CAD build for the part. Positions are in the model's coordinates, mm. A direction names the side the tool comes from. Coordinates: 2 decimals unless noted, no trailing zeros. Loops run counter-clockwise (first coordinate to the right, second up) from the corner with the lowest first, then second, coordinate; pieces in that order, holes last. Notation, with made-up numbers: (66, 58.25) -> (106, 58.25) arc R28 cw to (106, 89.25) -> close; hole circle Ø6 at (2.5, 24.5). An arc over 180 degrees is marked (long way). Write item = value, one per line. Start each with the question number.
(1) Pull direction Y, two halves, no side cores. Call faces 1 (the face through (-28.04, 6.07, -27.5)), 2 (the face through (0, 5, -22)), 3 (the face through (-12.8, 8, -22.2)), 4 (the face through (-2, 6, 0)): +Y half, -Y half, draft (parallel to the pull), parting line (faces both ways), or undercut.
(2) Band-saw the part on C-C (x = -24.5). Write the cut outline in (y, z), and give its area (3 significant figures).
(3) Band-saw the part on A-A (z = -31.4). Write the cut outline in (x, y).
(4) Band-saw the part on D-D (y = 6). Write the cut outline in (x, z), and give its area (3 significant figures).
(5) Band-saw the part on B-B (y = 3.5). Write the cut outline in (x, z), and give its area (3 significant figures).
(6) Flat gauge pins, fed straight in: P1, Ø7.5, axis at x = -25.5, z = -30.5, coming from the -Y side; P2, Ø0.9, axis at x = 0, z = -22.5, coming from the -Y side; P3, Ø1.6, axis at x = -27.5, y = 5, coming from the -Z side; P4, Ø3, axis at x = -25, z = -31.4, coming from the -Y side. Where does each tip first touch, or does it go through?
(7) Tool access for faces 5 (the face through (-27, 5, -28)), 6 (the face through (-0.5, 1.5, 0)), 7 (the face through (-21.5, 2, -29)): list every direction of +Z, -Z, +X, -X, +Y, -Y with a clear straight run to the whole face (end or side of a thin tool).
(8) Drill centre lines: line 1 (Z direction, x = -25, y = 1.7); line 2 (X direction, y = 1.55, z = 3); line 3 (Z direction, x = -19.5, y = 4). Where is each one in solid material? Low to high. Write a range as from..to.
Autodesk Inventor part; units mm, degrees
ref_plane "YZ Plane" through (0, 0, 0) normal (1, 0, 0) x (0, 1, 0)
ref_plane "XZ Plane" through (0, 0, 0) normal (0, 1, 0) x (-1, 0, 0)
ref_plane "XY Plane" through (0, 0, 0) normal (0, 0, 1) x (1, 0, 0)
sketch "Szkic1" plane through (0, 0, 0) normal (0, 1, 0) x (-1, 0, 0)
  line L0 (0, 0) -> (3, 0)
  line L1 (3, 0) -> (3, -25)
  line L2 (3, -25) -> (0, -25)
  line L3 (0, -25) -> (0, 0)
  line L4 (3, -25) -> (31, -25)
  line L5 (31, -25) -> (31, -22)
  line L6 (31, -22) -> (3, -22)
  line L7 (3, -22) -> (3, -25)
  point P0 (3, -22)
  dimension "d0" = 3
  dimension "d1" = 25
  dimension "d2" = 28
  dimension "d3" = 3
extrude "Wyciągnięcie proste1" add sketch "Szkic1" along normal blind 8
sketch "Szkic2" plane through (0, 0, 0) normal (1, 0, 0) x (0, 0, -1)
  line L0 (0, 0) -> (0, 8)
  line L1 (0, 8) -> (5, 8)
  line L2 (5, 8) -> (5, 0)
  line L3 (5, 0) -> (0, 0)
  line L4 (0, 0) -> (0, 8)
  dimension "d6" = 5
  dimension "d7" = 8
extrude "Wyciągnięcie proste2" add sketch "Szkic2" along normal blind 3
sketch "Szkic6" plane through (0, 8, 0) normal (0, 1, 0) x (1, 0, 0)
  line L0 (-31, 22) -> (-3, 22)
  line L1 (0, 25) -> (-31, 25)
  line L2 (-3, 22) -> (0, 22)
  line L3 (0, 22) -> (0, 25)
  line L4 (0, 25) -> (-3, 25)
  line L5 (-3, 25) -> (-3, 22)
  line L6 (-3, 25) -> (3, 25)
  line L7 (3, 25) -> (3, 19)
  line L8 (3, 19) -> (-3, 19)
  line L9 (-3, 19) -> (-3, 25)
  point P0 (0, 0)
  dimension "d19" = 6
  dimension "d20" = 6
extrude "Wyciągnięcie proste6" add sketch "Szkic6" against normal blind 8 contours L6 L7 L8 L9 L2 L3
sketch "Szkic7" plane through (0, 8, 0) normal (0, 1, 0) x (1, 0, 0)
  line L0 (3, 19) -> (3, 25)
  line L1 (-31, 25) -> (3, 25)
  line L2 (-3, 22) -> (-3, 0)
  circle A0 centre (0, 22) radius 1.5
  point P0 (0, 0)
  dimension "d23" = 3
  dimension "d42" = 3
  dimension "d43" = 3
extrude "Wyciągnięcie proste7" cut sketch "Szkic7" against normal blind 8
sketch "Szkic8" plane through (0, 8, 0) normal (0, 1, 0) x (1, 0, 0)
  circle A0 centre (0, 22) radius 1.5
  circle A1 centre (0, 22) radius 2
  point P0 (0, 0)
extrude "Wyciągnięcie proste8" add sketch "Szkic8" against normal blind 3 contours A0
sketch "Szkic9" plane through (0, 8, 0) normal (0, 1, 0) x (1, 0, 0)
  line L0 (-31, 25) -> (-31, 22)
  line L1 (3, 19) -> (3, 25)
  line L2 (-31, 25) -> (3, 25)
  line L3 (3, 25) -> (3, 24)
  line L4 (3, 24) -> (-31, 24)
  line L5 (-31, 24) -> (-31, 25)
  point P0 (0, 0)
  dimension "d28" = 1
extrude "Wyciągnięcie proste9" cut sketch "Szkic9" against normal blind 8
sketch "Szkic10" plane through (0, 0, -5) normal (0, 0, -1) x (-1, 0, 0)
  line L0 (0, 0) -> (0, 8)
  line L1 (-3, 8) -> (-3, 0)
  line L2 (0, 0) -> (-3, 0)
  line L3 (-3, 0) -> (-3, 8)
  line L4 (-3, 8) -> (0, 8)
  line L5 (0, 8) -> (0, 0)
  point P0 (-3, 0)
extrude "Wyciągnięcie proste10" cut sketch "Szkic10" against normal blind 3.7
sketch "Szkic11" plane through (0, 8, -19) normal (0, 0, 1) x (1, 0, 0)
  line L0 (-3, 0) -> (3, 0)
  line L1 (3, -8) -> (0, -8)
  line L2 (0, 0) -> (3, 0)
  line L3 (3, 0) -> (3, -8)
  line L4 (3, -8) -> (0, -8)
  line L5 (0, -8) -> (0, 0)
extrude "Wyciągnięcie proste11" cut sketch "Szkic11" against normal blind 0.5
sketch "Szkic12" plane through (3, 8, -24) normal (0, 0, -1) x (-1, 0, 0)
  line L0 (0, -8) -> (0, 0)
  line L1 (6, 0) -> (0, 0)
  line L2 (0, -8) -> (6, -8)
  line L3 (6, -8) -> (6, 0)
  line L4 (6, 0) -> (0, 0)
  line L5 (0, 0) -> (0, -8)
  point P0 (3, -8)
extrude "Wyciągnięcie proste12" add sketch "Szkic12" along normal blind 0.5
sketch "Szkic13" plane through (0, 0, -1.3) normal (1, 0, 0) x (0, 0, -1)
  line L0 (0, 0) -> (18.2, 0)
  line L1 (0, 8) -> (18.2, 8)
  line L2 (0, 0) -> (18.2, 0)
  line L3 (18.2, 0) -> (18.2, 8)
  line L4 (18.2, 8) -> (0, 8)
  line L5 (0, 8) -> (0, 0)
  point P0 (-1.3, 0)
  point P1 (18.2, 0)
extrude "Wyciągnięcie proste13" cut sketch "Szkic13" against normal blind 1
sketch "Szkic14" plane through (3, 8, -24.5) normal (0, 0, -1) x (-1, 0, 0)
  line L0 (4, 0) -> (0, 0)
  line L1 (6, -8) -> (6, 0)
  line L2 (0, 0) -> (6, 0)
  line L3 (6, 0) -> (6, -8)
  line L4 (6, -8) -> (0, -8)
  line L5 (0, -8) -> (0, 0)
  point P0 (3, -8)
extrude "Wyciągnięcie proste14" cut sketch "Szkic14" against normal blind 0.5
sketch "Szkic15" plane through (-3, 0, 0) normal (0, 0, 1) x (1, 0, 0)
  line L0 (6, 8) -> (6, 0)
  line L1 (0, 0) -> (0, 8)
  line L2 (6, 8) -> (0, 8)
  line L3 (0, 8) -> (0, 0)
  line L4 (0, 0) -> (6, 0)
  line L5 (6, 0) -> (6, 8)
  point P0 (3, 0)
extrude "Wyciągnięcie proste15" add sketch "Szkic15" along normal blind 4.7
sketch "Szkic16" plane through (3, 0, 0) normal (1, 0, 0) x (0, 0, -1)
  line L0 (-4.7, 8) -> (-4.7, 0)
  line L1 (1.3, 0) -> (1.3, 8)
  line L2 (-4.7, 0) -> (1.3, 0)
  line L3 (1.3, 0) -> (1.3, 8)
  line L4 (1.3, 8) -> (-4.7, 8)
  line L5 (-4.7, 8) -> (-4.7, 0)
  point P0 (0, 0)
extrude "Wyciągnięcie proste16" cut sketch "Szkic16" against normal blind 4
sketch "Szkic17" plane through (0, 8, 0) normal (0, 1, 0) x (1, 0, 0)
  line L0 (-1, 19.5) -> (-1, -4.7)
  line L1 (-3, -4.7) -> (-1, -4.7)
  line L2 (-1, -4.7) -> (-1, 0)
  line L3 (-1, 0) -> (-3, 0)
  line L4 (-3, 0) -> (-3, -4.7)
  line L5 (-3, 0) -> (3, 0)
  line L6 (3, 0) -> (3, -6)
  line L7 (3, -6) -> (-3, -6)
  line L8 (-3, -6) -> (-3, 0)
  point P0 (0, 0)
  dimension "d48" = 6
  dimension "d49" = 6
extrude "Wyciągnięcie proste17" cut sketch "Szkic17" against normal blind 5
sketch "Szkic18" plane through (0, 3, 0) normal (0, 1, 0) x (1, 0, 0)
  line L0 (-3, 0) -> (-1, 0)
  line L1 (-3, 0) -> (3, 0)
  line L2 (3, 0) -> (3, -6)
  line L3 (3, -6) -> (-3, -6)
  line L4 (-3, -6) -> (-3, 0)
  point P0 (0, 0)
  dimension "d52" = 6
  dimension "d53" = 6
extrude "Wyciągnięcie proste18" add sketch "Szkic18" against normal blind 3
sketch "Szkic19" plane through (0, 3, 0) normal (0, 1, 0) x (1, 0, 0)
  circle A0 centre (0, -3) radius 2
  line L0 (-3, -6) -> (-3, 0)
  line L1 (-3, -6) -> (3, -6)
  point P0 (0, 0)
  dimension "d56" = 4
  dimension "d57" = 3
  dimension "d58" = 3
extrude "Wyciągnięcie proste19" cut sketch "Szkic19" against normal blind 3
sketch "Szkic20" plane through (-31, 0, -22) normal (0, 0, 1) x (1, 0, 0)
  line L0 (34, 8) -> (0, 8)
  line L1 (0, 8) -> (7, 8)
  line L2 (7, 8) -> (7, 4)
  line L3 (7, 4) -> (0, 4)
  line L4 (0, 4) -> (0, 8)
  point P0 (31, 0)
  point P1 (7, 8)
  dimension "d61" = 7
  dimension "d62" = 4
extrude "Wyciągnięcie proste20" add sketch "Szkic20" along normal blind 4
sketch "Szkic21" plane through (-31, 0, -24) normal (-1, 0, 0) x (0, 0, 1)
  circle A0 centre (4, 6) radius 1.5
  line L0 (6, 8) -> (6, 4)
  line L1 (2, 4) -> (6, 4)
  point P0 (24, 0)
  point P1 (4, 4)
  dimension "d65" = 3
  dimension "d66" = 2
  dimension "d67" = 2
extrude "Wyciągnięcie proste21" cut sketch "Szkic21" against normal blind 6
sketch "Szkic22" plane through (3, 8, -24) normal (0, 0, -1) x (-1, 0, 0)
  line L0 (34, 0) -> (34, -8)
  line L1 (34, 0) -> (27, 0)
  line L2 (27, 0) -> (27, -4)
  line L3 (27, -4) -> (34, -4)
  line L4 (34, -4) -> (34, 0)
  point P0 (3, -8)
  dimension "d70" = 7
  dimension "d71" = 4
extrude "Wyciągnięcie proste22" add sketch "Szkic22" along normal blind 4
sketch "Szkic23" plane through (-31, 0, -24) normal (-1, 0, 0) x (0, 0, 1)
  circle A0 centre (-2, 6) radius 1.5
  line L0 (-4, 8) -> (6, 8)
  line L1 (-4, 4) -> (-4, 8)
  line L2 (2, 0) -> (2, 8)
  line L3 (6, 8) -> (2, 8)
  line L4 (2, 8) -> (2, 4)
  line L5 (2, 4) -> (6, 4)
  line L6 (6, 4) -> (6, 8)
  point P0 (24, 0)
  point P1 (-4, 6)
  dimension "d74" = 3
  dimension "d75" = 2
  dimension "d76" = 2
extrude "Wyciągnięcie proste23" cut sketch "Szkic23" against normal blind 7 contours L0 L6 L5 L2
extrude "Wyciągnięcie proste24" cut sketch "Szkic23" against normal blind 6 contours A0
sketch "Sketch24" plane through (3, 0, -24) normal (0, 0, -1) x (-1, 0, 0)
  line L0 (34, 4) -> (27, 4)
  line L1 (27, 4) -> (27, 8)
  line L2 (0, 8) -> (27, 8)
  line L3 (0, 0) -> (0, 8)
  line L4 (34, 0) -> (0, 0)
  line L5 (34, 4) -> (34, 0)
  point P0 (3, 0)
extrude "Extrusion25" add sketch "Sketch24" along normal blind 0.5
sketch "Szkic25" plane through (3, 0, -24.5) normal (0, 0, -1) x (-1, 0, 0)
  line L0 (27, 4) -> (34, 4)
  line L1 (27, 8) -> (27, 4)
  line L2 (27, 8) -> (0, 8)
  line L3 (0, 8) -> (0, 0)
  line L4 (0, 0) -> (34, 0)
  line L5 (34, 0) -> (34, 4)
  point P0 (3, 0)
extrude "Wyciągnięcie proste26" cut sketch "Szkic25" against normal blind 0.5
sketch "Szkic26" plane through (3, 0, -24) normal (0, 0, -1) x (-1, 0, 0)
  line L0 (34, 0) -> (6, 0)
  line L1 (34, 0) -> (24.5, 0)
  line L2 (24.5, 0) -> (24.5, 1.5)
  line L3 (24.5, 1.5) -> (34, 1.5)
  line L4 (34, 1.5) -> (34, 0)
  point P0 (3, 0)
  point P1 (24.5, 0)
  dimension "d85" = 9.5
  dimension "d86" = 1.5
extrude "Wyciągnięcie proste27" add sketch "Szkic26" along normal blind 10.5
sketch "Szkic27" plane through (-31, 1.5, -24) normal (0, 1, 0) x (1, 0, 0)
  circle A0 centre (6, 7.4) radius 1.55
  line L0 (7, 0) -> (0, 0)
  line L1 (0, 0) -> (0, 10.5)
  point P0 (31, -24)
  point P1 (0, 5.25)
  dimension "d89" = 3.1
  dimension "d90" = 7.4
  dimension "d91" = 6
extrude "Wyciągnięcie proste28" cut sketch "Szkic27" against normal blind 2
fillet "Fillet1" radius 3 2 edges at (3, 1.5, 0) (3, 1.5, 6)
fillet "Fillet2" radius 2 2 edges at (3, 4, -19.5) (3, 4, -24)
fillet "Zaokrąglenie3" radius 3 1 edges at (-3, 1.5, 6)
sketch "Szkic28" plane through (-31, 1.5, -24) normal (0, 1, 0) x (1, 0, 0)
  line L0 (0, -2) -> (28, -2)
  line L1 (0, 0) -> (0, 4)
  line L2 (7, 4) -> (0, 4)
  line L3 (7, 0) -> (7, 4)
  line L4 (7, 0) -> (0, 0)
  point P0 (31, -24)
extrude "Wyciągnięcie proste29" add sketch "Szkic28" along normal blind 2.5
sketch "Szkic29" plane through (-24, 1.5, -24) normal (0, 1, 0) x (1, 0, 0)
  line L0 (-7, 4) -> (0, 4)
  line L1 (0, 4) -> (0, 0)
  line L2 (2.5, 0) -> (0, 0)
  line L3 (2.5, 0) -> (2.5, 10.5)
  line L4 (-7, 10.5) -> (2.5, 10.5)
  line L5 (-7, 4) -> (-7, 10.5)
  circle A0 centre (-1, 7.4) radius 1.55
  point P0 (24, -24)
extrude "Wyciągnięcie proste30" add sketch "Szkic29" along normal blind 1
sketch "Szkic30" plane through (0, 0, 0) normal (0, -1, 0) x (1, 0, 0)
  line L0 (-24, -28) -> (-31, -28)
  line L1 (-24, -24) -> (-24, -28)
  line L2 (-21.5, -24) -> (-24, -24)
  line L3 (-21.5, -24) -> (-21.5, -34.5)
  line L4 (-21.5, -34.5) -> (-31, -34.5)
  line L5 (-31, -34.5) -> (-31, -28)
  circle A0 centre (-25, -31.4) radius 1.55
  point P0 (0, 0)
extrude "Wyciągnięcie proste31" cut sketch "Szkic30" against normal blind 1
sketch "Szkic31" plane through (0, 0, 0) normal (0, -1, 0) x (1, 0, 0)
  line L0 (-24, -24) -> (1, -24)
  line L1 (-31, -28) -> (-31, -22)
  line L2 (-24, -24) -> (-31, -24)
  line L3 (-31, -24) -> (-31, -25.3)
  line L4 (-31, -25.3) -> (-24, -25.3)
  line L5 (-24, -25.3) -> (-24, -24)
  line L6 (-24, -28) -> (-24, -24)
  line L7 (-24, -28) -> (-31, -28)
  line L8 (-31, -28) -> (-31, -25.3)
  line L9 (-31, -25.3) -> (-24, -25.3)
  line L10 (-24, -25.3) -> (-24, -28)
  point P0 (0, 0)
  dimension "d103" = 1.3
extrude "Wyciągnięcie proste32" cut sketch "Szkic31" against normal blind 1
properties part number "prawascianakolo" material "Tworzywo sztuczne PET"
Findings below:
q1.face_1 = undercut
q1.face_2 = -Y half
q1.face_3 = +Y half
q1.face_4 = draft
q2.outline = (0, -24) -> (1, -24) -> (1, -29.93) -> (2.5, -29.93) -> (2.5, -28) -> (8, -28) -> (8, -22) -> (0, -22) -> close; (1, -34.5) -> (2.5, -34.5) -> (2.5, -32.87) -> (1, -32.87) -> close
q2.area = 49.3 mm²
q3.outline = (-31, 1) -> (-26.55, 1) -> (-26.55, 2.5) -> (-31, 2.5) -> close; (-23.45, 1) -> (-21.5, 1) -> (-21.5, 2.5) -> (-23.45, 2.5) -> close
q4.outline = (-31, -28) -> (-24, -28) -> (-24, -24) -> (1, -24) arc R2 ccw to (3, -22) -> (3, -21.5) arc R2 ccw to (1, -19.5) -> (-1, -19.5) -> (-1, 0) -> (-3, 0) -> (-3, -22) -> (-31, -22) -> (-31, -24.5) -> (-25, -24.5) -> (-25, -27.5) -> (-31, -27.5) -> close
q4.area = 130 mm²
q5.outline = (-31, -28) -> (-24, -28) -> (-24, -24) -> (1, -24) arc R2 ccw to (3, -22) -> (3, -21.5) arc R2 ccw to (1, -19.5) -> (-1, -19.5) -> (-1, 0) -> (-3, 0) -> (-3, -22) -> (-31, -22) -> close; hole circle Ø3 at (0, -22)
q5.area = 141 mm²
q6.P1 = 1
q6.P2 = 5
q6.P3 = -28
q6.P4 = through
q7.face_5 = -Z, +X, -X, +Y
q7.face_6 = +X, +Y, -Y
q7.face_7 = -Z, +X, +Y, -Y
q8.line_1 = -34.5..-32.95, -29.85..-22
q8.line_2 = -3..-2, 2..3
q8.line_3 = -24..-22
